Autodesk Inventor part; units mm, degrees
ref_plane "YZ Plane" through (0, 0, 0) normal (1, 0, 0) x (0, 1, 0)
ref_plane "XZ Plane" through (0, 0, 0) normal (0, 1, 0) x (-1, 0, 0)
ref_plane "XY Plane" through (0, 0, 0) normal (0, 0, 1) x (1, 0, 0)
sketch "Boceto1" plane through (0, 0, 0) normal (0, 0, 1) x (1, 0, 0)
  circle A0 centre (0, 0) radius 125
  circle A1 centre (0, 0) radius 480
  dimension "d0" = 960
  dimension "d1" = 250
extrude "Extrusión1" add sketch "Boceto1" against normal blind 25
sketch "Boceto2" plane through (0, 0, 0) normal (0, 0, 1) x (1, 0, 0)
  circle A0 centre (0, 0) radius 340
  circle A1 centre (0, 0) radius 337
  dimension "d4" = 680
  dimension "d5" = 674
extrude "Extrusión2" cut sketch "Boceto2" against normal blind 5
sketch "Boceto3" plane through (0, 0, 0) normal (0, 0, 1) x (1, 0, 0)
  circle A0 centre (0, 0) radius 332.5 construction
  circle A1 centre (0, 332.5) radius 6
  circle A2 centre (-113.7217, 312.4478) radius 6
  circle A3 centre (-213.7269, 254.7098) radius 6
  circle A4 centre (-287.9534, 166.25) radius 6
  circle A5 centre (-327.4486, 57.738) radius 6
  circle A6 centre (-327.4486, -57.738) radius 6
  circle A7 centre (-287.9534, -166.25) radius 6
  circle A8 centre (-213.7269, -254.7098) radius 6
  circle A9 centre (-113.7217, -312.4478) radius 6
  circle A10 centre (0, -332.5) radius 6
  circle A11 centre (113.7217, -312.4478) radius 6
  circle A12 centre (213.7269, -254.7098) radius 6
  circle A13 centre (287.9534, -166.25) radius 6
  circle A14 centre (327.4486, -57.738) radius 6
  circle A15 centre (327.4486, 57.738) radius 6
  circle A16 centre (287.9534, 166.25) radius 6
  circle A17 centre (213.7269, 254.7098) radius 6
  circle A18 centre (113.7217, 312.4478) radius 6
  dimension "d8" = 665
  dimension "d9" = 12
  dimension "d12" = 360
extrude "Extrusión3" [suppressed]
properties part number "Brida_2 (flange_2) Lebus"
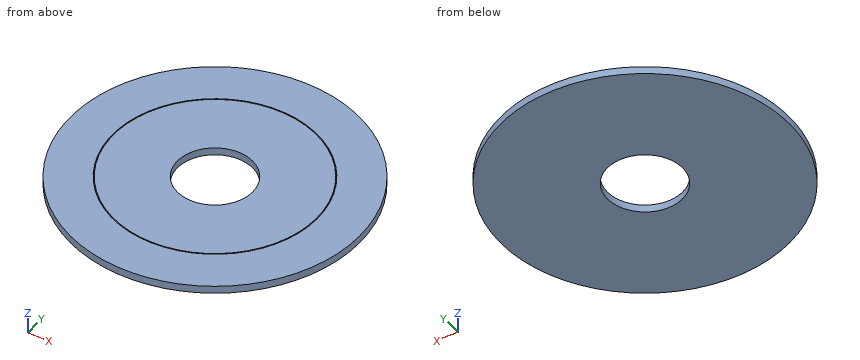
The listing builds one solid part. Answer for the finished solid, in the listing's coordinates (mm). Coordinates: 2 decimals unless noted, no trailing zeros. Loops run counter-clockwise (first coordinate to the right, second up) from the corner with the lowest first, then second, coordinate; pieces in that order, holes last. Notation, with made-up numbers: (72, 71) -> (115, 71) arc R15 ccw to (115, 83) -> close; hole circle Ø11 at (-21.5, 88). An arc over 180 degrees is marked (long way). Write item = value, one per line. Start each with the question number.
1) Given pin 1 Ø2 at (x, z) = (-129, -10.5) entering from +Y; pin 2 Ø5 at (y, z) = (-376, -17.5) entering from +X; pin 3 Ø3 at (y, z) = (305.5, -4) entering from -X, each flat-ended and moving along its own axis, determine where each tip first touches the part or whether it passes through.
2) A cutting plane is placed at A-A (x = 0). Give the vertices of the cut face in (y, z), then the cut area to 3 significant figures.
3) A cutting plane is placed at C-C (z = -20.5). Give the vertices of the cut face in (x, y), then the cut area to 3 significant figures.
4) Straight lines are drawn through the part: line 1 (Y direction, x = 0, z = -2.2); line 2 (Y direction, x = 0, z = -17.5); line 3 (X direction, y = 157.5, z = -3). For each, find the intervals that lie inside material, in ascending order. Write a range as from..to.
5) A cutting plane is placed at D-D (y = -201.5). Give the vertices of the cut face in (x, z), then the cut area to 3 significant figures.
Responses:
q1.pin_1 = 462.62
q1.pin_2 = 301.49
q1.pin_3 = -371.46
q2.outline = (-480, -25) -> (-125, -25) -> (-125, 0) -> (-337, 0) -> (-337, -5) -> (-340, -5) -> (-340, 0) -> (-480, 0) -> close; (125, -25) -> (480, -25) -> (480, 0) -> (340, 0) -> (340, -5) -> (337, -5) -> (337, 0) -> (125, 0) -> close
q2.area = 17,700 mm²
q3.outline = circle Ø960 at (0, 0); hole circle Ø250 at (0, 0)
q3.area = 675,000 mm²
q4.line_1 = -480..-340, -337..-125, 125..337, 340..480
q4.line_2 = -480..-125, 125..480
q4.line_3 = -453.42..-301.32, -297.93..297.93, 301.32..453.42
q5.outline = (-435.66, -25) -> (435.66, -25) -> (435.66, 0) -> (273.86, 0) -> (273.86, -5) -> (270.12, -5) -> (270.12, 0) -> (-270.12, 0) -> (-270.12, -5) -> (-273.86, -5) -> (-273.86, 0) -> (-435.66, 0) -> close
q5.area = 21,700 mm²
